from build123d import *

# Parameters (mm, degrees)
SKETCH1_R                = 5.5
BOSS_EXTRUDE1_DEPTH      = 1.25
SKETCH2_R                = 3.75
CUT_EXTRUDE1_DEPTH       = 1.25
BOSS_EXTRUDE6_DEPTH      = 1.25
SKETCH6_W                = 4.926299948
SKETCH6_H                = 1.5
BOSS_EXTRUDE7_DEPTH      = 15
SKETCH8_R                = 6
BOSS_EXTRUDE8_DEPTH      = 1.25
SKETCH9_R                = 3.75
CUT_EXTRUDE3_DEPTH       = 1.25
BOSS_EXTRUDE9_DEPTH      = 4.75
BOSS_EXTRUDE9_DEPTH_BACK = 1.25
SKETCH10_W               = 4.888756282
SKETCH10_H               = 10
SKETCH11_R               = 1.669068308
CUT_EXTRUDE4_DEPTH       = 10
SKETCH12_R               = 1.5
CUT_EXTRUDE5_DEPTH       = 10
SKETCH13_R               = 1.5
CUT_EXTRUDE6_DEPTH       = 10


with BuildPart() as part:
    # Sketch1 → Boss-Extrude1 (new body)
    with BuildSketch(Plane(origin=(0, 0, 0), x_dir=(1, 0, 0), z_dir=(0, 1, 0))):
        with Locations(Location((0, 0, 0), (0, 0, 270))):
            Circle(SKETCH1_R)
    extrude(amount=BOSS_EXTRUDE1_DEPTH)

    # Sketch2 → Cut-Extrude1 (cut)
    with BuildSketch(Plane(origin=(0, 1.25, 0), x_dir=(1, 0, 0), z_dir=(0, 1, 0))):
        with Locations(Location((0, 0, 0), (0, 0, 270))):
            Circle(SKETCH2_R)
    extrude(amount=-CUT_EXTRUDE1_DEPTH, mode=Mode.SUBTRACT)

    # Sketch3 → Boss-Extrude6 (add)
    with BuildSketch(Plane(origin=(0, 1.25, 0), x_dir=(1, 0, 0), z_dir=(0, 1, 0))):
        Polygon((-2.5, 3.749893265), (0, 3.749893265), (2.426299948, 3.749893265), (2.426299948, 27.250106735), (-2.5, 27.250106735), align=None)
        Polygon((-1.997595264, -4.040063509), (-3.247595264, -1.875), (-4.49106014, 0.278744342), (-24.842657128, -11.471255658), (-22.349192253, -15.790063509), align=None)
        Polygon((4.497595264, 0.290063509), (3.247595264, -1.875), (1.99170365, -4.050268084), (22.343300639, -15.800268084), (24.849192253, -11.459936491), align=None)
    extrude(amount=-BOSS_EXTRUDE6_DEPTH)

    # Sketch6 → Boss-Extrude7 (add)
    with BuildSketch(Plane(origin=(0, 1.25, 0), x_dir=(1, 0, 0), z_dir=(0, 1, 0))):
        with Locations((-0.036850026, 5.250106735)):
            Rectangle(SKETCH6_W, SKETCH6_H)
        Polygon((-6.169311431, -0.690194493), (-3.675846556, -5.009002344), (-2.37680845, -4.259002344), (-4.870273325, 0.059805507), align=None)
        Polygon((3.974013034, -5.181148841), (6.474013034, -0.851021822), (5.174974928, -0.101021822), (2.674974928, -4.431148841), align=None)
    extrude(amount=BOSS_EXTRUDE7_DEPTH)

    # Sketch8 → Boss-Extrude8 (add)
    with BuildSketch(Plane(origin=(0, 16.25, 0), x_dir=(1, 0, 0), z_dir=(0, 1, 0))):
        with Locations(Location((0, 0, 0), (0, 0, 66.147511133))):
            Circle(SKETCH8_R)
    extrude(amount=BOSS_EXTRUDE8_DEPTH)

    # Sketch9 → Cut-Extrude3 (cut)
    with BuildSketch(Plane(origin=(0, 17.5, 0), x_dir=(1, 0, 0), z_dir=(0, 1, 0))):
        with Locations(Location((0, 0, 0), (0, 0, 270))):
            Circle(SKETCH9_R)
    extrude(amount=-CUT_EXTRUDE3_DEPTH, mode=Mode.SUBTRACT)

    # Sketch10 → Boss-Extrude9 (add, two sides: drawn at the far end of the back side and taken through both)
    with BuildSketch(Plane(origin=(0, 1.25, 0), x_dir=(1, 0, 0), z_dir=(0, 1, 0)).offset(-BOSS_EXTRUDE9_DEPTH_BACK)):
        Polygon((-31.069234844, -20.686506698), (-22.408980806, -15.686506698), (-24.782868576, -11.57481247), (-33.443122613, -16.57481247), align=None)
        with Locations((-0.036850026, 32.250106735)):
            Rectangle(SKETCH10_W, SKETCH10_H)
        Polygon((31.044029351, -20.730163892), (22.383775314, -15.730163892), (24.808717579, -11.530040683), (33.468971617, -16.530040683), align=None)
    extrude(amount=BOSS_EXTRUDE9_DEPTH + BOSS_EXTRUDE9_DEPTH_BACK)

    # Sketch11 → Cut-Extrude4 (cut)
    with BuildSketch(Plane(origin=(-32.259446291, 0, 18.625), x_dir=(0.5000000000000004, 0, 0.8660254037844385), z_dir=(-0.8660254037844384, 0, 0.5000000000000003))):
        with Locations((0.006535125, 3)):
            Circle(SKETCH11_R)
    extrude(amount=-CUT_EXTRUDE4_DEPTH, mode=Mode.SUBTRACT)

    # Sketch12 → Cut-Extrude5 (cut)
    with BuildSketch(Plane(origin=(0, 0, -37.250106735), x_dir=(-1, 0, 0), z_dir=(0, 0, -1))):
        with Locations((0.018425013, 3)):
            Circle(SKETCH12_R)
    extrude(amount=-CUT_EXTRUDE5_DEPTH, mode=Mode.SUBTRACT)

    # Sketch13 → Cut-Extrude6 (cut)
    with BuildSketch(Plane(origin=(32.259446291, 0, 18.625), x_dir=(0.4999999999999998, 0, -0.8660254037844388), z_dir=(0.8660254037844388, 0, 0.4999999999999998))):
        with Locations((-0.005891614, 3)):
            Circle(SKETCH13_R)
    extrude(amount=-CUT_EXTRUDE6_DEPTH, mode=Mode.SUBTRACT)


solid = part.part
Geometry check sheet. Reference: the model listing, model coordinates, mm. A direction names the side the tool comes from. Give positions to 0.01 mm unless a question says otherwise; leave off trailing zeros. Order: outer loops, then holes, each group sorted by start corner. A loop starts at its lowest first (then second) coordinate and runs counter-clockwise, first axis right, second up. Notation, with made-up numbers: (21.5, 56) - (72.5, 56) arc R31 ccw to (72.5, 90) - close; hole circle Ø2 at (14, -15). An arc over 180 degrees is marked (long way). Use one line per item in the form item = value.
1) Sectioned sample at D-D (y = 3). Count the separate pieces of the cut face and the enclosed holes in it, and give its area (3 significant figures).
Working result:
separate_pieces = 9
enclosed_holes = 0
area = 73.9 mm^2
2) Draft check along Z on faces 1 (the face through (5.207, 8.645, 3.046)), 2 (the face through (0, 1.25, -17)), 3 (the face through (1, 17.5, 4)). Enter one of: released by +Z, released by -Z, zero draft, split by the parting line, or undercut.
Working result:
face_1 = released by +Z
face_2 = undercut
face_3 = zero draft
3) Sectioned sample at A-A (y = 8.5). Record the boundary of the cut face in (x, z).
Working result:
outline = (-6.17, 0.69) - (-4.87, -0.06) - (-2.38, 4.26) - (-3.68, 5.01) - close; (-2.5, -6) - (2.43, -6) - (2.43, -4.5) - (-2.5, -4.5) - close; (2.67, 4.43) - (5.17, 0.1) - (6.47, 0.85) - (3.97, 5.18) - close
4) Depth check by flat-ended pin: pin 1 Ø10 at (x, z) = (-11, -5) entering from +Y; pin 2 Ø1.5 at (x, y) = (0.5, 7.5) entering from +Z; pin 3 Ø1.5 at (x, z) = (-0.5, -30) entering from +Y; pin 4 Ø2 at (x, z) = (13, 5.5) entering from +Y. Enter the tip coordinate at first touch or a pass-through.
Working result:
pin_1 = through
pin_2 = -4.5
pin_3 = 6
pin_4 = 1.25
5) Access from +Z, -Z, +X, -X, +Y, -Y to the whole of each face (thin tool, end or side, straight path). Record for faces 4 (the face through (-2.481, 3, -32)), 5 (the face through (-5.5, 16.9, 2.4)), 6 (the face through (0, 6, -32)).
Working result:
face_4 = -Z, -X, +Y, -Y
face_5 = +Y
face_6 = -Z, +X, -X, +Y
6) Sectioned sample at B-B (z = 2.5). Record the boundary of the cut face in (x, y), and give its area (3 significant figures).
Working result:
outline = (-9.3, 0) - (-2.8, 0) - (-2.8, 1.25) - (-3.39, 1.25) - (-3.39, 16.25) - (-2.8, 16.25) - (-2.8, 17.5) - (-5.45, 17.5) - (-5.45, 16.25) - (-5.12, 16.25) - (-5.12, 1.25) - (-9.3, 1.25) - close; (2.8, 0) - (9.33, 0) - (9.33, 1.25) - (5.52, 1.25) - (5.52, 16.25) - (5.45, 16.25) - (5.45, 17.5) - (2.8, 17.5) - (2.8, 16.25) - (3.79, 16.25) - (3.79, 1.25) - (2.8, 1.25) - close
area = 74.9 mm^2
7) Sectioned sample at C-C (z = -17). Record the boundary of the cut face in (x, y), and give its area (3 significant figures).
Working result:
outline = (-2.5, 0) - (2.43, 0) - (2.43, 1.25) - (-2.5, 1.25) - close
area = 6.16 mm^2
8) Material ranges on probe 1 along X at (y, z) = (16.8, 0); probe 2 along Y at (x, z) = (-2, -14); probe 3 along Z at (x, y) = (1, 11.5), recorded low to high. Write a range as from..to.
Working result:
probe_1 = -6..-3.75, 3.75..6
probe_2 = 0..1.25
probe_3 = -6..-4.5
